Answer from the drawing. Dimensions are ordinates in mm from the lowest x, y and z of the part. A direction names the side the tool comes from. Round coordinates to 2 decimals unless told otherwise and drop trailing zeros. Write each loop counter-clockwise with the first axis right and the second up, starting at its lowest first coordinate (ties: lowest second). Pieces come first, ordered by that corner, then holes. Notation, with made-up numbers: (-21, -2) - (-7, -2) arc R28 cw to (-7, 31) - close; hole circle Ø11 at (38.25, -9.75). An arc over 180 degrees is marked (long way). Answer as a JSON object with one key per item and string values.
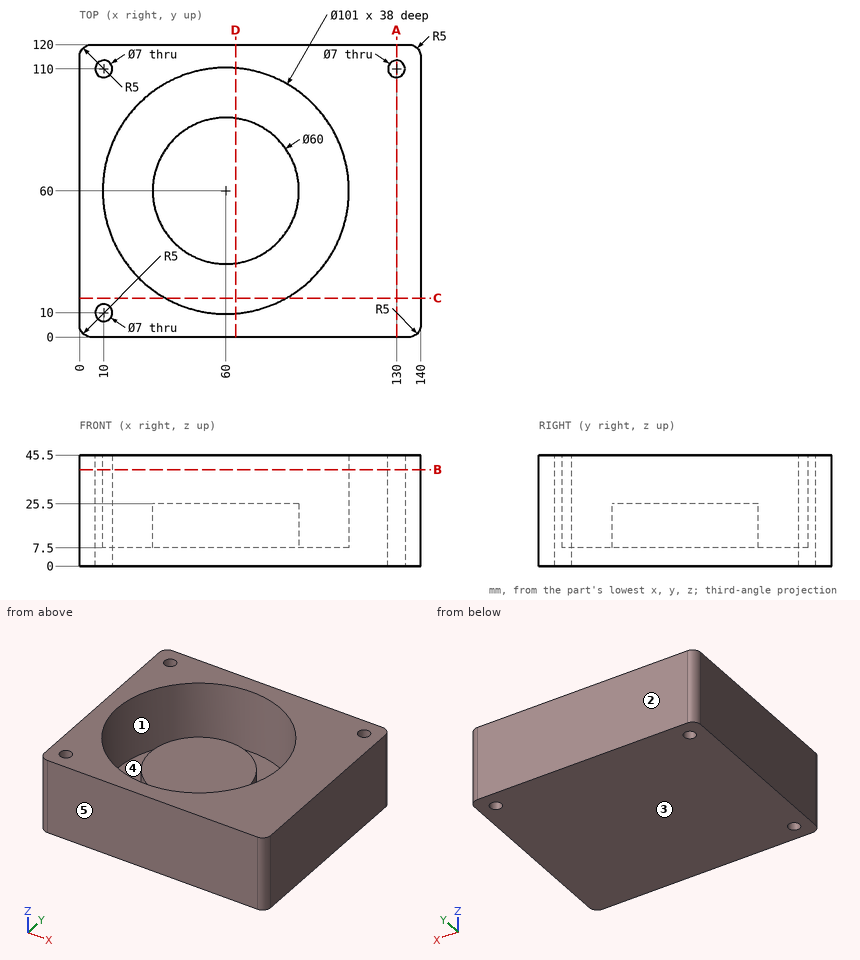
Item 1: Determine the mould class of the marked faces 1, 2 and 3 for opening direction Y: pulls with the +Y half, pulls with the -Y half, needs draft (parallel to the pull), parting line crosses it, or undercut.
Results found:
{"face 1": "undercut", "face 2": "pulls with the +Y half", "face 3": "needs draft"}
Item 2: Consider line 1 along Y through (x, z) = (60, 24); line 2 along X through (y, z) = (82, 24); line 3 along X through (y, z) = (66, 18.5). Determine where each line is inside the solid, lowest interval first.
Results found:
{"line 1": "0 to 9.5, 30 to 90, 110.5 to 120", "line 2": "0 to 14.54, 39.6 to 80.4, 105.46 to 140", "line 3": "0 to 9.86, 30.61 to 89.39, 110.14 to 140"}
Item 3: For the marked faces 4 and 5, determine the directions among +Z, -Z, +X, -X, +Y, -Y from which every point of the face is accessible in a straight line to the end or side of a thin tool.
Results found:
{"face 4": "+Z", "face 5": "+Z, -Z, +X, -X, -Y"}
Item 4: Each of these flat-tipped pins is pushed along its axis until it touches: P1, Ø2, axis at x = 80, y = 55.5, coming from the +Z side; P2, Ø1.5, axis at x = 34.5, y = 20, coming from the +Z side; P3, Ø6.5, axis at x = 10, y = 10, coming from the +Z side. Where does it stop, or does it pass through?
Results found:
{"P1": "z = 25.5", "P2": "z = 7.5", "P3": "through"}
Item 5: A cutting plane is placed at C-C (y = 16). Write down the section's boundary in (x, z).
Results found:
{"outline": "(0, 0) - (140, 0) - (140, 45.5) - (84.78, 45.5) - (84.78, 7.5) - (35.22, 7.5) - (35.22, 45.5) - (0, 45.5) - close"}
Item 6: A cutting plane is placed at A-A (x = 130). Write down the section's boundary in (y, z).
Results found:
{"outline": "(0, 0) - (106.5, 0) - (106.5, 45.5) - (0, 45.5) - close; (113.5, 0) - (120, 0) - (120, 45.5) - (113.5, 45.5) - close"}
Item 7: A cutting plane is placed at B-B (z = 39.5). Write down the section's boundary in (x, y), and give its area (3 significant figures).
Results found:
{"outline": "(0, 5) arc R5 ccw to (5, 0) - (135, 0) arc R5 ccw to (140, 5) - (140, 115) arc R5 ccw to (135, 120) - (5, 120) arc R5 ccw to (0, 115) - close; hole circle Ø7 at (10, 10); hole circle Ø7 at (10, 110); hole circle Ø101 at (60, 60); hole circle Ø7 at (130, 110)", "area": "8,650 mm²"}
Item 8: A cutting plane is placed at D-D (x = 64). Write down the section's boundary in (y, z), and give its area (3 significant figures).
Results found:
{"outline": "(0, 0) - (120, 0) - (120, 45.5) - (110.34, 45.5) - (110.34, 7.5) - (89.73, 7.5) - (89.73, 25.5) - (30.27, 25.5) - (30.27, 7.5) - (9.66, 7.5) - (9.66, 45.5) - (0, 45.5) - close", "area": "2,700 mm²"}
